Part model, mm, in its own coordinate system. Face numbers are marked on the shaded views. A direction names the side the tool comes from. Give positions to 0.01 mm unless a question says otherwise; leave off trailing zeros. Write each loop counter-clockwise with the first axis right and the second up, starting at its lowest first coordinate (ties: lowest second). Pieces come first, ordered by that corner, then holes. Notation, with made-up numbers: M 47.25,-18 L 105.25,-18 A16 cw 105.25,-13 Z; hole C 87.25,-25.75 d8. An arc over 180 degrees is marked long. Use CSV: the item, a comma, the result in double quotes. Start each with the question number.
Item 1: Cut at D-D (x = 53.5). List the corners of the cut face in (y, z) (3 decimals).
Item 2: Drill centre lines: line 1 (Z direction, x = 0, y = 31.5) (1 decimal); line 2 (Y direction, x = -21, z = -31) (3 decimals); line 3 (Y direction, x = 17, z = 14.5) (1 decimal). Where is each one in solid material? Low to high. Write a range as [from, to].
Item 3: Pin check, flat tips, straight feed: pin 1 (6 mm diameter, centred on x = -13, y = 42.5, fed in from +Z); pin 2 (5 mm diameter, centred on y = 24.5, z = 14.5, fed in from -X); pin 3 (4 mm diameter, centred on y = 17, z = -1, fed in from -X) (3 decimals). Stop position of each tip, or through.
Item 4: Mould opens along Z. For the marked faces 1, 2 and 3 say: released by +Z, released by -Z, zero draft, split by the parting line, or undercut.
Item 5: Cut at A-A (x = 0). Count the separate pieces of the cut face and the enclosed holes in it, then the cut area to 3 significant figures.
Item 6: Cut at C-C (y = 3). List the corners of the cut face in (x, z) (1 decimal), then the cut area to 3 significant figures.
Item 7: Which spindle directions (+Z, -Z, +X, -X, +Y, -Y) get a long thin tool onto all of the face, cutting with end or side? Do the marked faces 4, 5 and 6. Say none if no direction does.
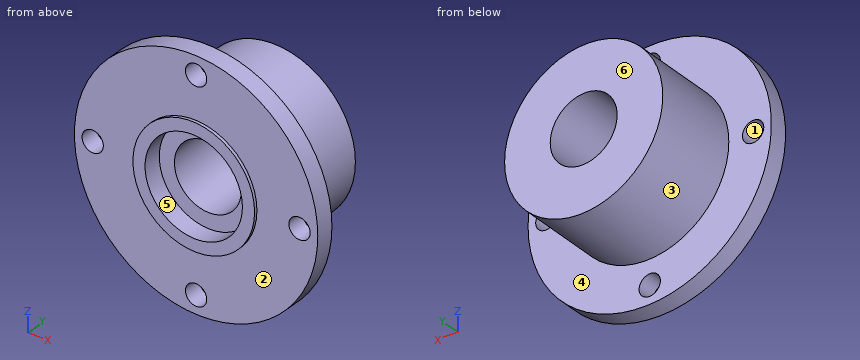
from build123d import *

# Parameters (mm, degrees)
F0_R             = 63.5
F1_DEPTH         = 9.525
F2_R             = 31.75
F3_DEPTH         = 1.5875
F4_R             = 25.4
F5_DEPTH         = 9.525
F6_R             = 41.275
F7_DEPTH         = 44.45
F8_R             = 17.4625
F9_DEPTH         = 55.5635
F10_R            = 5.55625
F11_DEPTH        = 53.976
F11_COPIES_COUNT = 4


# Not quite as in the source:
# - a pattern or mirror of a feature is missing from the dataset's text; its kind, count and spacing are read off the source's solid


with BuildPart() as f1:
    # F0 (on Front) → F1 (new body)
    with BuildSketch(Plane.XZ):
        Circle(F0_R)
    extrude(amount=-F1_DEPTH)

    # F2 (on face) → F3 (join)
    with BuildSketch(Plane.XZ):
        Circle(F2_R)
    extrude(amount=F3_DEPTH)

    # F4 (on face) → F5 (cut)
    with BuildSketch(Plane.XZ.offset(1.5875)):
        Circle(F4_R)
    extrude(amount=-F5_DEPTH, mode=Mode.SUBTRACT)

    # F6 (on face) → F7 (join)
    with BuildSketch(Plane(origin=(0, 9.525, 0), x_dir=(-1, 0, 0), z_dir=(0, 1, 0))):
        Circle(F6_R)
    extrude(amount=F7_DEPTH)

    # F8 (on face) → F9 (cut, through all)
    with BuildSketch(Plane.XZ.offset(1.5875)):
        Circle(F8_R)
    extrude(amount=-F9_DEPTH, mode=Mode.SUBTRACT)

    # F10 (on face) → F11 (cut, through all)
    with BuildSketch(Plane.XZ):
        with Locations((53.975, 0)):
            Circle(F10_R)
    f11 = extrude(amount=-F11_DEPTH, mode=Mode.SUBTRACT)

    # F11_copies: F11 ×4 about axis
    f11_copies_axis = Axis((0, 0, 0), (0, 1, 0))
    for i in range(1, F11_COPIES_COUNT):
        add(f11.rotate(f11_copies_axis, i * 360 / F11_COPIES_COUNT), mode=Mode.SUBTRACT)


solid = f1.part
Worked answers:
1,outline,"M 0,-34.205 L 9.525,-34.205 L 9.525,-5.536 L 0,-5.536 Z; M 0,5.536 L 9.525,5.536 L 9.525,34.205 L 0,34.205 Z"
2,line 1,"z = [-41.3, -17.5], [17.5, 41.3]"
2,line 2,"y = [0, 53.975]"
2,line 3,"y = [7.9, 54]"
3,pin 1,"stops at z = 40.05"
3,pin 2,"stops at x = -39.49"
3,pin 3,"stops at x = -41.275"
4,face 1,"undercut"
4,face 2,"zero draft"
4,face 3,"split by the parting line"
5,separate pieces,"4"
5,enclosed holes,"0"
5,area,"2,680 mm^2"
6,outline,"C 0,0 d127; hole C -54,0 d11.1; hole C 0,0 d50.8; hole C 0,-54 d11.1; hole C 0,54 d11.1; hole C 54,0 d11.1"
6,area,"10,300 mm^2"
7,face 4,"+Y"
7,face 5,"-Y"
7,face 6,"+Z, -Z, +X, -X, +Y"
